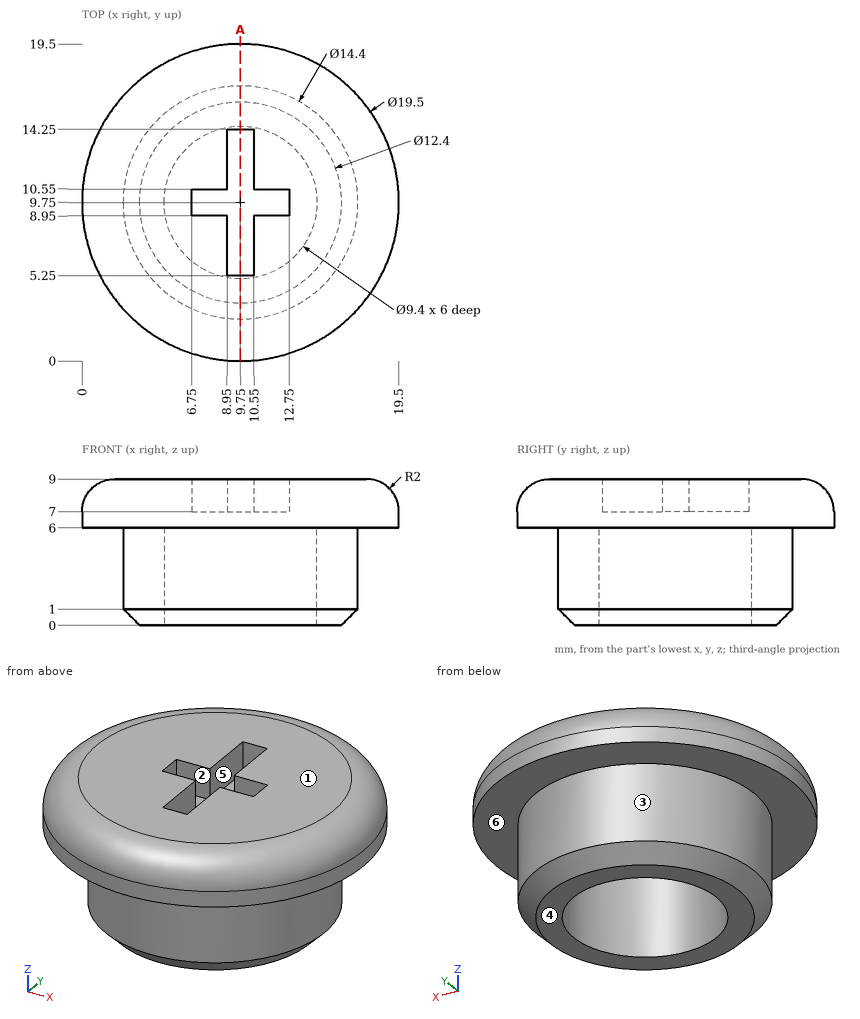
Could you check a few things on this drawing? It's one solid part, dimensions in mm from its lowest x, y, z. A direction names the side the tool comes from. Round coordinates to 2 decimals unless told otherwise and drop trailing zeros. Order: outer loops, then holes, each group sorted by start corner. A loop starts at its lowest first (then second) coordinate and runs counter-clockwise, first axis right, second up. Notation, with made-up numbers: M 88,-20 L 99,-20 A13 cw 99,-1 Z; hole C 81.5,88.5 d10. An arc over 180 degrees is marked long. Return JSON: item names as keys, results as strings. Group by question number.
1. If we section it at A-A on x = 9.75: List the corners of the cut face in (y, z) for me, then the cut area to 3 significant figures.
2. If we mould it in two halves opening along Y, with no side actions, what happens to the marked faces 1, 2 and 3? For each: pulls with the +Y half, pulls with the -Y half, needs draft (parallel to the pull), parting line crosses it, or undercut.
3. Please list where these lines run through material, in increasing order: probe 1 along Y at (x, z) = (9.75, 2.05); probe 2 along Z at (x, y) = (11.75, 9.75); probe 3 along Z at (x, y) = (7, 13.5).
4. I'm going to push flat-ended pins straight in: pin 1 Ø8.5 at (x, y) = (9.75, 9.75) entering from +Z; pin 2 Ø5 at (x, z) = (2, 2.5) entering from -Y; pin 3 Ø5 at (x, z) = (2.5, 6) entering from -Y; pin 4 Ø2 at (x, z) = (11, 8) entering from -Y. Where does each tip first touch, or does it pass through?
5. On a 3-axis mill with a long thin cutter (end or side, diameter ignored), from which of +Z, -Z, +X, -X, +Y, -Y can I reach the whole of each face in a straight line? I mean the marked faces 4, 5 and 6. Say none if no direction works.
Reply:
{
 "1": {"outline": "M 0,6 L 2.55,6 L 2.55,1 L 3.55,0 L 5.05,0 L 5.05,6 L 14.45,6 L 14.45,0 L 15.95,0 L 16.95,1 L 16.95,6 L 19.5,6 L 19.5,7 A2 ccw 17.5,9 L 14.25,9 L 14.25,7 L 5.25,7 L 5.25,9 L 2,9 A2 ccw 0,7 Z", "area": "67.8 mm^2"},
 "2": {"face 1": "needs draft", "face 2": "undercut", "face 3": "parting line crosses it"},
 "3": {"probe 1": "2.55 to 5.05, 14.45 to 16.95", "probe 2": "6 to 7", "probe 3": "6 to 9"},
 "4": {"pin 1": "z = 9", "pin 2": "y = 4.82", "pin 3": "y = 1.24", "pin 4": "y = 0.03"},
 "5": {"face 4": "-Z, +X, -X, +Y, -Y", "face 5": "+Z", "face 6": "-Z"}
}
